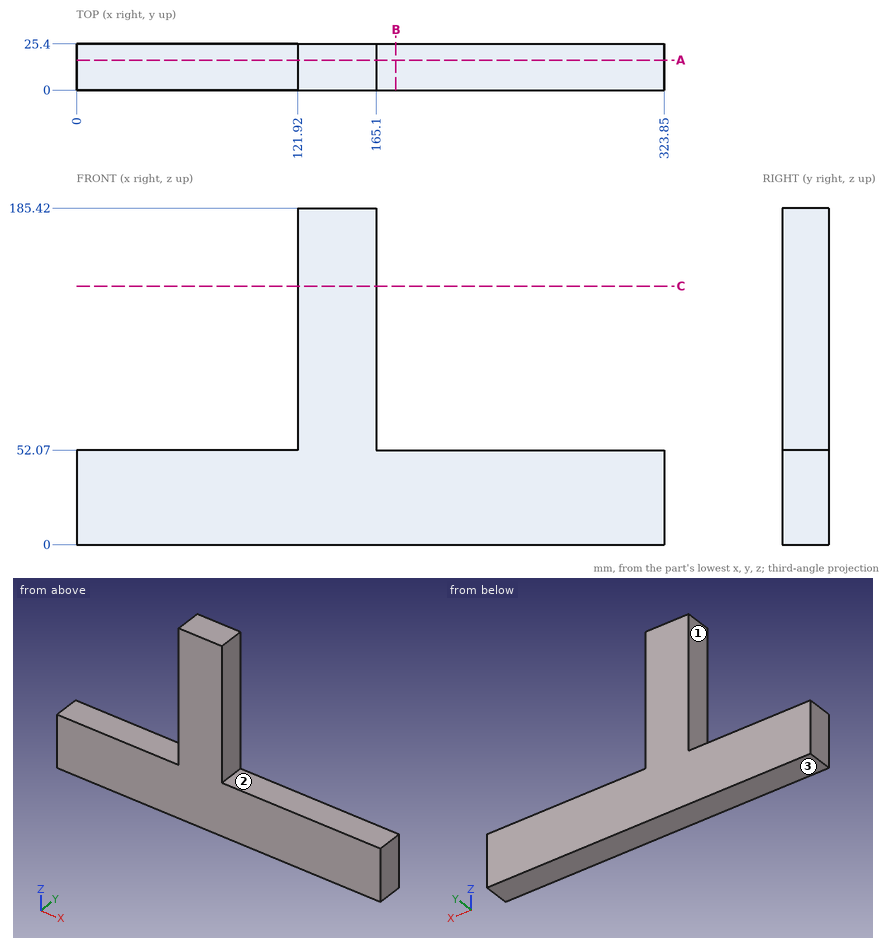
The drawing under review shows one solid part. Ordinate dimensions are in mm from its lowest x, y, z. A direction names the side the tool comes from. Coordinates: 2 decimals unless noted, no trailing zeros. Write each loop counter-clockwise with the first axis right and the second up, starting at its lowest first coordinate (ties: lowest second). Pieces come first, ordered by that corner, then holes. Notation, with made-up numbers: (39, 42.5) - (69, 42.5) arc R22 cw to (69, 69.5) - close; hole circle Ø10 at (43, -15.5). An arc over 180 degrees is marked (long way). Answer as CSV lines item,"result".
(1) We need section C-C (z = 142.5). Give the boundary of the cut face in (x, y).
Data:
outline,"(121.92, 0) - (165.1, 0) - (165.1, 25.4) - (121.92, 25.4) - close"
(2) Clearance check with flat-ended pins moving along their axes: pin 1 Ø7.5 at (y, z) = (14, 124) entering from -X; pin 2 Ø12.5 at (x, y) = (72, 13) entering from +Z; pin 3 Ø8 at (y, z) = (20, 79.5) entering from +X. State where each tip first meets the part, or that it passes through.
Data:
pin 1,"stops at x = 121.92"
pin 2,"stops at z = 52.07"
pin 3,"stops at x = 165.1"
(3) We need section A-A (y = 16.5). Give the boundary of the cut face in (x, z).
Data:
outline,"(0, 0) - (323.85, 0) - (323.85, 52.07) - (165.1, 52.07) - (165.1, 185.42) - (121.92, 185.42) - (121.92, 52.07) - (0, 52.07) - close"
(4) Tool access review of the marked faces 1, 2 and 3: name each direction out of +Z, -Z, +X, -X, +Y, -Y from which nothing blocks a thin tool from reaching the whole face with its end or side.
Data:
face 1,"+Z, -X, +Y, -Y"
face 2,"+Z, +X, +Y, -Y"
face 3,"-Z, +X, -X, +Y, -Y"
(5) For line 1 along X through (y, z) = (21.25, 72.5); line 2 along Z through (x, y) = (268, 2), list the stretches that pass through material, from the lowest coordinate up. Write a range as [from, to].
Data:
line 1,"x = [121.92, 165.1]"
line 2,"z = [0, 52.07]"
(6) We need section B-B (x = 176). Give the boundary of the cut face in (y, z), plus the area to 3 significant figures.
Data:
outline,"(0, 0) - (25.4, 0) - (25.4, 52.07) - (0, 52.07) - close"
area,"1,320 mm2"
